Source: three-view drawing plus pictorial views. Frame: mm from the lowest corner of the part. A direction names the side the tool comes from. Give positions to 0.01 mm unless a question says otherwise; leave off trailing zeros. Order: outer loops, then holes, each group sorted by start corner. A loop starts at its lowest first (then second) coordinate and runs counter-clockwise, first axis right, second up. Notation, with made-up numbers: M -29,16 L 12,16 A20 cw 12,41 Z; hole C -9,-33.75 d11. An arc over 180 degrees is marked long. Use CSV: the item, a comma, the result in double quotes. Start each with the question number.
1. Pin query (flat end, axial travel): P1, Ø3.5, axis at x = 20.1, y = 24.8, coming from the -Z side; P2, Ø1.5, axis at x = 9.5, z = 26.5, coming from the -Y side; P3, Ø2.5, axis at x = 39.9, y = 5, coming from the +Z side. Return the tip coordinate at first contact, or that it passes through.
2. Section query A-A, the plane y = 5. Return the cut outline in (x, z), plus the area to 3 significant figures.
3. Section query D-D, the plane y = 19.5. Return the cut outline in (x, z).
4. Section query B-B, the plane z = 25. Return the cut outline in (x, y), plus the area to 3 significant figures.
5. Reachability of the marked faces 1 and 2 from +Z, -Z, +X, -X, +Y, -Y: full face, straight path, thin tool, end or side. Return the list, or none.
6. Line query: line 1 along Y through (x, z) = (30, 38.8); line 2 along Z through (x, y) = (13, 3). Output: solid intervals per line, ascending. Write a range as [from, to].
7. Section query C-C, the plane x = 26. Return the cut outline in (y, z).
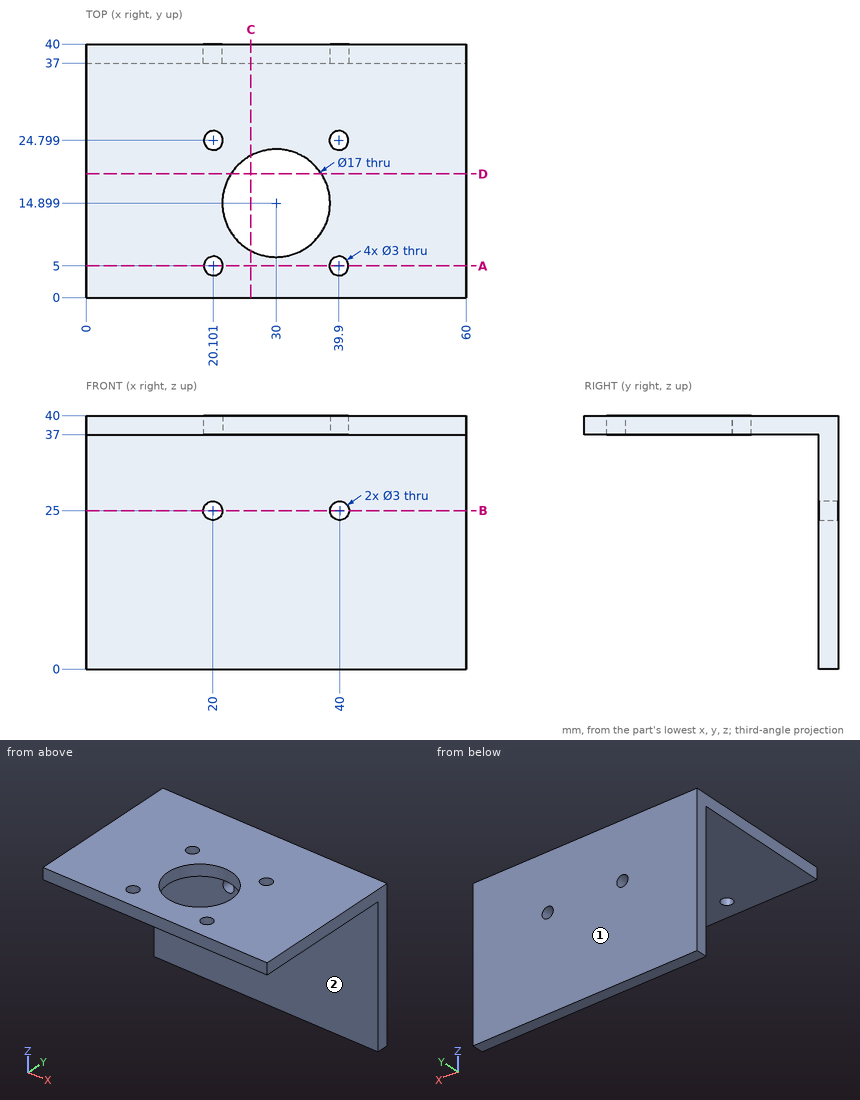
Result set:
1,P1,"z = 37"
1,P2,"y = 37"
1,P3,"through"
2,outline,"M 0,37 L 18.6,37 L 18.6,40 L 0,40 Z; M 21.6,37 L 38.4,37 L 38.4,40 L 21.6,40 Z; M 41.4,37 L 60,37 L 60,40 L 41.4,40 Z"
2,area,"162 mm2"
3,outline,"M 0,37 L 22.85,37 L 22.85,40 L 0,40 Z; M 37.15,37 L 60,37 L 60,40 L 37.15,40 Z"
4,outline,"M 0,37 L 18.5,37 L 18.5,40 L 0,40 Z; M 21.5,37 L 38.5,37 L 38.5,40 L 21.5,40 Z; M 41.5,37 L 60,37 L 60,40 L 41.5,40 Z"
4,area,"162 mm2"
5,face 1,"+Z, -Z, +X, -X, +Y"
5,face 2,"-Z, +X, -X, -Y"
6,line 1,"[0, 6.4], [23.4, 40]"
6,line 2,"[37, 40]"
7,outline,"M 0,37 L 7.4,37 L 7.4,40 L 0,40 Z; M 22.4,37 L 37,37 L 37,0 L 40,0 L 40,40 L 22.4,40 Z"
